For this review, take the finished solid that the model builds, in its own axes (mm). Give positions to 0.01 mm unless a question says otherwise; leave off trailing zeros. Order: outer loops, then holes, each group sorted by start corner. A loop starts at its lowest first (then second) coordinate and runs counter-clockwise, first axis right, second up.
Item 1: Consider section B-B (x = 11). Give the boundary of the cut face in (y, z) (3 decimals), plus the area to 3 significant figures.
Item 2: For probe 1 along X at (y, z) = (19, 2.9); probe 2 along Y at (x, z) = (18.5, 2.6); probe 3 along X at (y, z) = (-3, 1.95), list the stretches that pass through material, from the lowest coordinate up.
Item 3: For P1, Ø1.6, axis at x = -12.5, z = 1, coming from the -Y side; P2, Ø1, axis at x = 19, z = 2, coming from the +Y side; P3, Ø1, axis at y = -19, z = 1.5, coming from the +X side, all flat-tipped, find the tip position at first contact; note any pin that passes through.
Item 4: Consider section A-A (y = 17). Give the boundary of the cut face in (x, z) (3 decimals), plus the area to 3 significant figures.
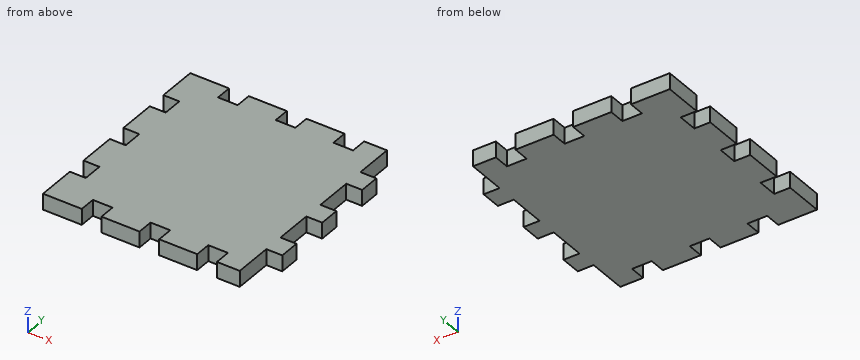
```python
from build123d import *

# Parameters (mm, degrees)
BOSS_EXTRUDE1_DEPTH = 3.175
BOSS_EXTRUDE2_DEPTH = 3.175


with BuildPart() as part:
    # Sketch2 → Boss-Extrude1 (new body)
    with BuildSketch(Plane.XY):
        Polygon((-2, 17.975), (-2, 21.15), (-9.5, 21.15), (-9.5, 17.975), (-13.5, 17.975), (-13.5, 21.15), (-21.15, 21.15), (-21.15, 13.5), (-17.975, 13.5), (-17.975, 9.5), (-21.15, 9.5), (-21.15, 2), (-17.975, 2), (-17.975, -2), (-21.15, -2), (-21.15, -9.5), (-17.975, -9.5), (-17.975, -13.5), (-21.15, -13.5), (-21.15, -21.15), (-13.5, -21.15), (-13.5, -17.975), (-9.5, -17.975), (-9.5, -21.15), (-2, -21.15), (-2, -17.975), (2, -17.975), (2, -21.15), (9.5, -21.15), (9.5, -17.975), (13.5, -17.975), (13.5, -21.15), (17.975, -21.15), (17.975, -13.5), (21.15, -13.5), (21.15, -9.5), (17.975, -9.5), (17.975, -2), (21.15, -2), (21.15, 2), (17.975, 2), (17.975, 9.5), (21.15, 9.5), (21.15, 13.5), (17.975, 13.5), (17.975, 21.15), (13.5, 21.15), (13.5, 17.975), (9.5, 17.975), (9.5, 21.15), (2, 21.15), (2, 17.975), align=None)
    extrude(amount=BOSS_EXTRUDE1_DEPTH)

    # Sketch3 → Boss-Extrude2 (add)
    with BuildSketch(Plane.XY.offset(3.175)):
        Polygon((18.01564, -2.04064), (21.19064, -2.04064), (21.19064, 2.04064), (18.01564, 2.04064), (18.01564, 9.45936), (21.19064, 9.45936), (21.19064, 13.54064), (18.01564, 13.54064), (18.01564, 21.19064), (13.45936, 21.19064), (13.45936, 18.01564), (9.54064, 18.01564), (9.54064, 21.19064), (1.95936, 21.19064), (1.95936, 18.01564), (-1.95936, 18.01564), (-1.95936, 21.19064), (-9.54064, 21.19064), (-9.54064, 18.01564), (-13.45936, 18.01564), (-13.45936, 21.19064), (-21.19064, 21.19064), (-21.19064, 13.45936), (-18.01564, 13.45936), (-18.01564, 9.54064), (-21.19064, 9.54064), (-21.19064, 1.95936), (-18.01564, 1.95936), (-18.01564, -1.95936), (-21.19064, -1.95936), (-21.19064, -9.54064), (-18.01564, -9.54064), (-18.01564, -13.45936), (-21.19064, -13.45936), (-21.19064, -21.19064), (-13.45936, -21.19064), (-13.45936, -18.01564), (-9.54064, -18.01564), (-9.54064, -21.19064), (-1.95936, -21.19064), (-1.95936, -18.01564), (1.95936, -18.01564), (1.95936, -21.19064), (9.54064, -21.19064), (9.54064, -18.01564), (13.45936, -18.01564), (13.45936, -21.19064), (18.01564, -21.19064), (18.01564, -13.54064), (21.19064, -13.54064), (21.19064, -9.45936), (18.01564, -9.45936), align=None)
    extrude(amount=-BOSS_EXTRUDE2_DEPTH)


solid = part.part
```
Resolved:
1. outline: (-18.016, 0) - (18.016, 0) - (18.016, 3.175) - (-18.016, 3.175) - close
1. area: 114 mm2
2. probe 1: x = -21.19 to -13.46, -9.54 to -1.96, 1.96 to 9.54, 13.46 to 18.02
2. probe 2: y = -13.54 to -9.46, -2.04 to 2.04, 9.46 to 13.54
2. probe 3: x = -21.19 to 18.02
3. P1: stops at y = -18.02
3. P2: stops at y = 13.54
3. P3: stops at x = 18.02
4. outline: (-21.191, 0) - (18.016, 0) - (18.016, 3.175) - (-21.191, 3.175) - close
4. area: 124 mm2
